from build123d import *

# Parameters (mm, degrees)
SKETCH1_W           = 101.6
SKETCH1_H           = 127
BOSS_EXTRUDE2_DEPTH = 88.9
SKETCH3_R           = 39.6875
BOSS_EXTRUDE3_DEPTH = 161.925
SKETCH4_R           = 6.35
BOSS_EXTRUDE4_DEPTH = 25.4
SKETCH5_R           = 7.9375
BOSS_EXTRUDE5_DEPTH = 38.1
SKETCH6_R           = 3.96875
CUT_EXTRUDE1_DEPTH  = 25.4


with BuildPart() as part:
    # Sketch1 → Boss-Extrude2 (new body)
    with BuildSketch(Plane(origin=(0, 0, 0), x_dir=(1, 0, 0), z_dir=(0, 1, 0))):
        Rectangle(SKETCH1_W, SKETCH1_H)
    extrude(amount=BOSS_EXTRUDE2_DEPTH)

    # Sketch3 → Boss-Extrude3 (add)
    with BuildSketch(Plane(origin=(0, 88.9, 0), x_dir=(1, 0, 0), z_dir=(0, 1, 0))):
        Circle(SKETCH3_R)
    extrude(amount=BOSS_EXTRUDE3_DEPTH)

    # Sketch4 → Boss-Extrude4 (add)
    with BuildSketch(Plane(origin=(0, 250.825, 0), x_dir=(1, 0, 0), z_dir=(0, 1, 0))):
        Circle(SKETCH4_R)
    extrude(amount=BOSS_EXTRUDE4_DEPTH)

    # Sketch5 → Boss-Extrude5 (add)
    with BuildSketch(Plane(origin=(0, 0, 0), x_dir=(-1, 0, 0), z_dir=(0, -1, 0))):
        with Locations((0, -22.225)):
            Circle(SKETCH5_R)
    extrude(amount=BOSS_EXTRUDE5_DEPTH)

    # Sketch6 → Cut-Extrude1 (cut)
    with BuildSketch(Plane(origin=(0, 0, 0), x_dir=(-1, 0, 0), z_dir=(0, -1, 0))):
        with Locations((42.8625, -38.1)):
            Circle(SKETCH6_R)
        with Locations((-42.8625, -38.1)):
            Circle(SKETCH6_R)
        with Locations((42.8625, 50.174061918)):
            Circle(SKETCH6_R)
        with Locations((-42.8625, 50.174061918)):
            Circle(SKETCH6_R)
    extrude(amount=-CUT_EXTRUDE1_DEPTH, mode=Mode.SUBTRACT)


solid = part.part
Read the model definition and answer for the solid it produces. Units are mm, in the model's axes. A direction names the side the tool comes from. Coordinates: 2 decimals unless noted, no trailing zeros. Order: outer loops, then holes, each group sorted by start corner. A loop starts at its lowest first (then second) coordinate and runs counter-clockwise, first axis right, second up. Notation, with made-up numbers: M 34,-28.5 L 58,-28.5 A31 ccw 58,8.5 Z; hole C 52,13.5 d4. An arc over 180 degrees is marked long. Put each result on its own line as item: value. Start each with the question number.
Item 1: Section C-C, the plane y = 210 is taken. Determine the outline of the cut face in (x, z) (1 decimal).
Item 2: For faces 4 (the face through (43, 25.4, 38)), 5 (the face through (37.855, 168.729, -11.921)), 6 (the face through (-1, 44, 63.5)), determine the directions among +Z, -Z, +X, -X, +Y, -Y from which every point of the face is accessible in a straight line to the end or side of a thin tool.
Item 3: Section D-D, the plane z = -22.5 is taken. Determine the outline of the cut face in (x, y) (3 decimals).
Item 4: Given pin 1 Ø5 at (x, z) = (42.86, -50.17) entering from +Y; pin 2 Ø12 at (y, z) = (148.5, -23.5) entering from -X; pin 3 Ø12 at (x, y) = (20, 230.5) entering from +Z, each flat-ended and moving along its own axis, determine where each tip first touches the part or whether it passes through.
Item 5: The mould has two halves that part along X. Classify faces 1 (the face through (-39.94, 12.52, -52.86)), 2 (the face through (50.8, 44, 1)), 3 (the face through (1.721, -18.783, 29.974)): +X half, -X half, draft (parallel to the pull), parting line (faces both ways), or undercut.
Item 6: Consider probe 1 along Y at (x, z) = (15, -52); probe 2 along Y at (x, z) = (-4, 24) (3 decimals); probe 3 along Z at (x, y) = (36.5, 125.5). Determine where each line is inside the solid, lowest interval first. Write a range as [from, to].
Computed:
1. outline: C 0,0 d79.4
2. face 4: -Y
2. face 5: +Y
2. face 6: +Z, +X, -X, +Y, -Y
3. outline: M -50.8,0 L 50.8,0 L 50.8,88.9 L 32.693,88.9 L 32.693,250.825 L -32.693,250.825 L -32.693,88.9 L -50.8,88.9 Z
4. pin 1: stops at y = 88.9
4. pin 2: stops at x = -35.62
4. pin 3: stops at z = 37.14
5. face 1: undercut
5. face 2: +X half
5. face 3: parting line
6. probe 1: y = [0, 88.9]
6. probe 2: y = [-38.1, 250.825]
6. probe 3: z = [-15.58, 15.58]
